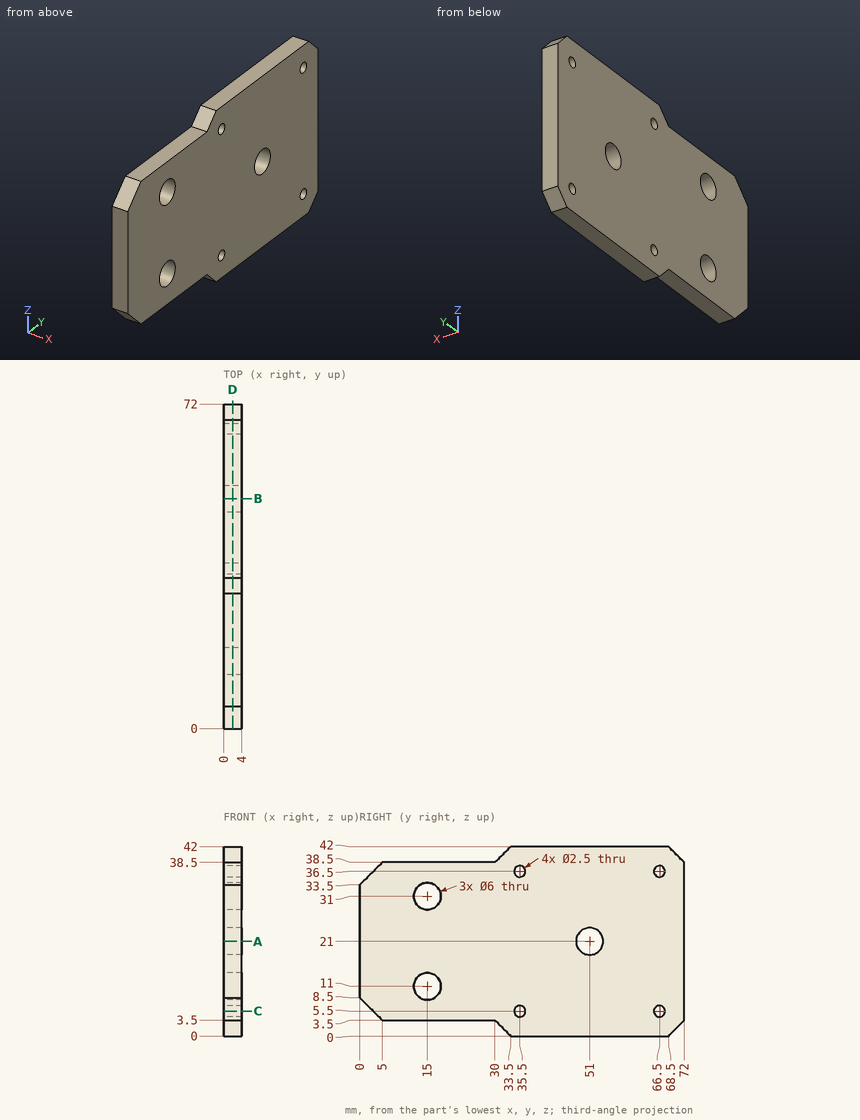
The figure shows three views and two pictorial views of one solid part (mm, origin at its lowest corner). Answer the questions. Coordinates: 2 decimals unless noted, no trailing zeros. Order: outer loops, then holes, each group sorted by start corner. A loop starts at its lowest first (then second) coordinate and runs counter-clockwise, first axis right, second up.
Q1. A cutting plane is placed at B-B, the plane y = 51. Write down the section's boundary in (x, z), and give its area (3 significant figures).
Q2. A cutting plane is placed at D-D, the plane x = 2. Write down the section's boundary in (y, z), and give its area (3 significant figures).
Q3. Given P1, Ø2, axis at y = 66.5, z = 5.5, coming from the +X side (1 decimal); P2, Ø8, axis at y = 15, z = 11, coming from the -X side; P3, Ø1.2, axis at x = 1, y = 21, coming from the +Z side; P4, Ø2, axis at x = 2.5, y = 16.5, coming from the -Z side, each flat-ended and moving along its own axis, determine where each tip first touches the part or whether it passes through.
Q4. A cutting plane is placed at A-A, the plane z = 21. Write down the section's boundary in (x, y), and give its area (3 significant figures).
Q5. A cutting plane is placed at C-C, the plane z = 5.5. Write down the section's boundary in (x, y), and give its area (3 significant figures).
Q6. Consider line 1 (Z direction, x = 2, y = 66.5); line 2 (Y direction, x = 2.1, z = 11); line 3 (Z direction, x = 1.4, y = 15). Determine where each line is inside the solid, lowest interval first.
Answers follow:
1. outline: (0, 0) - (4, 0) - (4, 18) - (0, 18) - close; (0, 24) - (4, 24) - (4, 42) - (0, 42) - close
1. area: 144 mm2
2. outline: (0, 8.5) - (5, 3.5) - (30, 3.5) - (33.5, 0) - (68.5, 0) - (72, 3.5) - (72, 38.5) - (68.5, 42) - (33.5, 42) - (30, 38.5) - (5, 38.5) - (0, 33.5) - close; hole circle Ø6 at (15, 11); hole circle Ø6 at (15, 31); hole circle Ø2.5 at (35.5, 5.5); hole circle Ø2.5 at (35.5, 36.5); hole circle Ø6 at (51, 21); hole circle Ø2.5 at (66.5, 5.5); hole circle Ø2.5 at (66.5, 36.5)
2. area: 2,660 mm2
3. P1: passes through
3. P2: stops at x = 0
3. P3: stops at z = 38.5
3. P4: stops at z = 3.5
4. outline: (0, 0) - (4, 0) - (4, 48) - (0, 48) - close; (0, 54) - (4, 54) - (4, 72) - (0, 72) - close
4. area: 264 mm2
5. outline: (0, 3) - (4, 3) - (4, 34.25) - (0, 34.25) - close; (0, 36.75) - (4, 36.75) - (4, 65.25) - (0, 65.25) - close; (0, 67.75) - (4, 67.75) - (4, 72) - (0, 72) - close
5. area: 256 mm2
6. line 1: z = 0 to 4.25, 6.75 to 35.25, 37.75 to 42
6. line 2: y = 0 to 12, 18 to 72
6. line 3: z = 3.5 to 8, 14 to 28, 34 to 38.5
